Geometry check sheet. Reference: the model listing, model coordinates, mm. Give positions to 0.01 mm unless a question says otherwise; leave off trailing zeros. Loops run counter-clockwise (first coordinate to the right, second up) from the corner with the lowest first, then second, coordinate; pieces in that order, holes last. Notation, with made-up numbers: (62.25, -38.75) -> (101.25, -38.75) arc R20 ccw to (101.25, -33.75) -> close; hole circle Ø10 at (47, 1.5). An arc over 180 degrees is marked (long way). Answer in a Markdown table with one row per item. Add a question column.
```python
from build123d import *

# Parameters (mm, degrees)
F0_W     = 60.7525799423
F0_H     = 66.2546996027
F2_R     = 25.4
F3_DEPTH = 127


with BuildPart() as f1:
    # F0 (on Front) → F1 (revolve)
    with BuildSketch(Plane.XZ):
        with Locations((1.3755289838, 3.4388257191)):
            Rectangle(F0_W, F0_H)
    revolve(axis=Axis((1.3755289838, 0, 36.5661755204), (1, 0, 0)))

    # F2
    f2_edges = [f1.edges().sort_by_distance(p)[0] for p in [
        (31.751819, 0, 102.820875),
        (-29.000761, 0, 102.820875),
    ]]
    fillet(f2_edges, radius=F2_R)

    # F3 (cut): a face of the model
    f3_faces = [f1.faces().sort_by_distance(p)[0] for p in [
        (31.7518189549, 0, 36.5661755204),
    ]]
    extrude(f3_faces, amount=-F3_DEPTH, mode=Mode.SUBTRACT)


solid = f1.part
```
1. Gauge pin test, flat ends, axial feed: pin 1 Ø1 at (x, y) = (-12, -12.5) entering from -Z; pin 2 Ø6 at (x, z) = (9, 87.5) entering from -Y; pin 3 Ø10 at (x, y) = (-18, -11.5) entering from -Z. Record the tip position at first contact, or that the pin passes through.
2. Sectioned sample at C-C (x = 19). Enter the section's corners in (y, z), plus the area to 3 significant figures.
3. Release check for a two-part mould opening along Y. For faces 1 (the face through (1.445, 2.913, 102.757)), 2 (the face through (1.801, 12.272, -2.402)) record: released by +Y, released by -Y, zero draft, split by the parting line, or undercut.
4. Sectioned sample at A-A (y = 0). Enter the section's corners in (x, z).
5. Material ranges on L1, parallel to Z at x = -16, y = 9; L2, parallel to Z at x = 27.5, y = -18; L3, parallel to Y at x = -23.5, z = 22.5, recorded low to high. Write a range as from..to.
6. Sectioned sample at B-B (x = 12). Enter the section's corners in (y, z), plus the area to 3 significant figures.
Response:
| question | item | result |
|---|---|---|
| 1 | pin 1 | stops at z = -27.24 |
| 1 | pin 2 | stops at y = -45.57 |
| 1 | pin 3 | stops at z = -27.01 |
| 2 | outline | circle Ø125.76 at (0, 36.57); hole circle Ø81.71 at (0, 36.57) |
| 2 | area | 7,180 mm2 |
| 3 | face 1 | split by the parting line |
| 3 | face 2 | undercut |
| 4 | outline | (-29, -4.29) arc R25.4 ccw to (-3.6, -29.69) -> (6.35, -29.69) arc R25.4 ccw to (31.75, -4.29) -> close; (-29, 77.42) -> (31.75, 77.42) arc R25.4 ccw to (6.35, 102.82) -> (-3.6, 102.82) arc R25.4 ccw to start |
| 5 | L1 | z = -25.81..-3.28, 76.42..98.94 |
| 5 | L2 | z = -15.32..-0.11, 73.24..88.46 |
| 5 | L3 | y = -54.87..-38.36, 38.36..54.87 |
| 6 | outline | circle Ø131.24 at (0, 36.57); hole circle Ø81.71 at (0, 36.57) |
| 6 | area | 8,280 mm2 |
